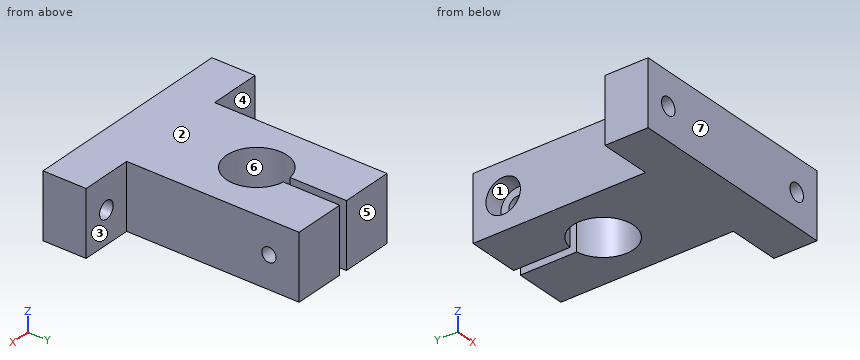
from build123d import *

# Parameters (mm, degrees)
BOSS_EXTRUDE1_DEPTH                                = 15
SKETCH5_R                                          = 2
CUT_EXTRUDE3_DEPTH                                 = 15
CHAMBRAGE_POUR_VIS_T_TE_HEXAGONALE_M41_D           = 4.3
CHAMBRAGE_POUR_VIS_T_TE_HEXAGONALE_M41_DEPTH       = 12
CHAMBRAGE_POUR_VIS_T_TE_HEXAGONALE_M41_CBORE_D     = 8
CHAMBRAGE_POUR_VIS_T_TE_HEXAGONALE_M41_CBORE_DEPTH = 4.4
TROU_TARAUD_M41_D                                  = 3.3


with BuildPart() as part:
    # Sketch1 → Boss-Extrude1 (new body)
    with BuildSketch(Plane.XY):
        with BuildLine():
            Line((-26, 0), (-26, -40))
            Line((-26, -40), (-38, -40))
            Line((-38, -40), (-38, -50))
            Line((-38, -50), (12, -50))
            Line((12, -50), (12, -40))
            Line((12, -40), (0, -40))
            Line((0, -40), (0, 0))
            Line((0, 0), (-12, 0))
            Line((-12, 0), (-12, -13.07179677))
            ThreePointArc((-12, -13.07179677), (-13, -27), (-14, -13.07179677))
            Line((-14, -13.07179677), (-14, 0))
            Line((-14, 0), (-26, 0))
        make_face()
    extrude(amount=BOSS_EXTRUDE1_DEPTH)

    # Sketch5 → Cut-Extrude3 (cut)
    with BuildSketch(Plane(origin=(0, -40, 0), x_dir=(1, 0, 0), z_dir=(0, 1, 0))):
        with Locations(Location((6, -7.5, 0), (0, 0, 270))):
            Circle(SKETCH5_R)
        with Locations(Location((-32, -7.5, 0), (0, 0, 270))):
            Circle(SKETCH5_R)
    extrude(amount=-CUT_EXTRUDE3_DEPTH, mode=Mode.SUBTRACT)

    # Chambrage pour vis à tête hexagonale M41
    with Locations(Plane.ZY.offset(26)):
        with Locations((7.569852971, -7)):
            CounterBoreHole(CHAMBRAGE_POUR_VIS_T_TE_HEXAGONALE_M41_D / 2, CHAMBRAGE_POUR_VIS_T_TE_HEXAGONALE_M41_CBORE_D / 2, CHAMBRAGE_POUR_VIS_T_TE_HEXAGONALE_M41_CBORE_DEPTH, depth=CHAMBRAGE_POUR_VIS_T_TE_HEXAGONALE_M41_DEPTH)

    # Trou taraudé M41 (through all)
    with Locations(Plane(origin=(0, 0, 0), x_dir=(0, 0, -1), z_dir=(1, 0, 0))):
        with Locations((-7.5, -7)):
            Hole(TROU_TARAUD_M41_D / 2)


solid = part.part
Can you work these out from the model? Positions are in its coordinate system, mm. Face numbers are marked on the shaded views. A direction names the side the tool comes from. Coordinates: 2 decimals unless noted, no trailing zeros. Write each loop counter-clockwise with the first axis right and the second up, starting at its lowest first coordinate (ties: lowest second). Pieces come first, ordered by that corner, then holes. Notation, with made-up numbers: M 66,-36 L 102,-36 A32 cw 102,-6 Z; hole C 4.25,77 d4. An arc over 180 degrees is marked long. Use one line per item in the form item = value.
Q1. If we section it at A-A (x = 6): Write out the boundary of the cut face in (y, z), then the cut area to 3 significant figures.
Model answer:
outline = M -50,0 L -40,0 L -40,5.5 L -50,5.5 Z; M -50,9.5 L -40,9.5 L -40,15 L -50,15 Z
area = 110 mm^2
Q2. If we section it at C-C (z = 7.5): State how many separate pieces and enclosed holes the cut face has, then the cut area to 3 significant figures.
Model answer:
separate_pieces = 5
enclosed_holes = 0
area = 1,170 mm^2
Q3. If we section it at D-D (x = -10): Write out the boundary of the cut face in (y, z), then the cut area to 3 significant figures.
Model answer:
outline = M -50,0 L -26.32,0 L -26.32,15 L -50,15 Z; M -13.68,0 L 0,0 L 0,15 L -13.68,15 Z; hole C -7,7.5 d3.3
area = 552 mm^2
Q4. We'd pull the mould along Y, two halves only. Please class the marked faces 5, 6 and 7: +Y half, -Y half, draft (parallel to the pull), parting line (faces both ways), or undercut.
Model answer:
face_5 = +Y half
face_6 = undercut
face_7 = -Y half
Q5. For the marked faces 1, 2, 3 and 4, which set-ups out of +Z, -Z, +X, -X, +Y, -Y let a thin tool reach every point of the face, with its end or its side?
Model answer:
face_1 = -X
face_2 = +Z, +X, -X, +Y, -Y
face_3 = +Z, -Z, +X, +Y
face_4 = +Z, -Z, -X, +Y
Q6. I need wall thicknesses on line 1 along X through (y, z) = (-44.75, 7.5); line 2 along X through (y, z) = (-8, 12.25); line 3 along Y through (x, z) = (-3, 7.5). Which ranges of each line are inside material? Lowest first, please. Write a range as from..to.
Model answer:
line_1 = -38..-34, -30..4, 8..12
line_2 = -26..-14, -12..0
line_3 = -50..-8.65, -5.35..0
Q7. For P1, Ø8, axis at y = -9, z = 10, coming from the -X side; P2, Ø4, axis at y = -7, z = 7.57, coming from the +X side; P3, Ø3.5, axis at x = 6, z = 7.5, coming from the +Y side; P4, Ø6, axis at x = 7, z = 9.5, coming from the +Y side, each with a flat end and sliding along its axis, tell me the tip position at first contact or that it passes through.
Model answer:
P1 = -26
P2 = 0
P3 = through
P4 = -40
Q8. If we section it at B-B (y = -20): Write out the boundary of the cut face in (x, z), then the cut area to 3 significant figures.
Model answer:
outline = M -26,0 L -20,0 L -20,15 L -26,15 Z; M -6,0 L 0,0 L 0,15 L -6,15 Z
area = 180 mm^2
